from build123d import *

# Parameters (mm, degrees)
SKETCH1_W           = 200
SKETCH1_H           = 150
BOSS_EXTRUDE1_DEPTH = 30
FILLET1_R           = 20
FILLET2_R           = 10
SKETCH2_W           = 15
SKETCH2_H           = 15
CUT_EXTRUDE1_DEPTH  = 183.756668825
FILLET4_R           = 5
SKETCH3_R           = 5
BOSS_EXTRUDE2_DEPTH = 20


with BuildPart() as part:
    # Sketch1 → Boss-Extrude1 (new body)
    with BuildSketch(Plane(origin=(0, 0, 0), x_dir=(1, 0, 0), z_dir=(0, 1, 0))):
        Rectangle(SKETCH1_W, SKETCH1_H)
    extrude(amount=BOSS_EXTRUDE1_DEPTH)

    # Fillet1
    fillet1_edges = [part.edges().sort_by_distance(p)[0] for p in [
        (0, 30, 75),
    ]]
    fillet(fillet1_edges, radius=FILLET1_R)

    # Fillet2
    fillet2_edges = [part.edges().sort_by_distance(p)[0] for p in [
        (100, 30, -10),
        (100, 5, 75),
        (100, 24.142135624, 69.142135624),
        (-100, 5, 75),
        (-100, 24.142135624, 69.142135624),
        (-100, 30, -10),
    ]]
    fillet(fillet2_edges, radius=FILLET2_R)

    # Sketch2 → Cut-Extrude1 (cut, through all)
    with BuildSketch(Plane.XY.offset(75)):
        with Locations((0, 7.5)):
            Rectangle(SKETCH2_W, SKETCH2_H)
    extrude(amount=-CUT_EXTRUDE1_DEPTH, mode=Mode.SUBTRACT)

    # Fillet4
    fillet4_edges = [part.edges().sort_by_distance(p)[0] for p in [
        (-7.5, 0, 0),
        (7.5, 0, 0),
    ]]
    fillet(fillet4_edges, radius=FILLET4_R)

    # Sketch3 → Boss-Extrude2 (add)
    with BuildSketch(Plane(origin=(0, 30, 0), x_dir=(1, 0, 0), z_dir=(0, 1, 0))):
        with Locations(Location((30, 5, 0), (0, 0, 270))):
            Circle(SKETCH3_R)
    boss_extrude2 = extrude(amount=BOSS_EXTRUDE2_DEPTH)

    # Mirror1: Boss-Extrude2 across plane
    add(boss_extrude2.mirror(Plane(origin=(0, 0, 0), x_dir=(0, 0, 1), z_dir=(1, 0, 0))))


solid = part.part
Here's how the part is built. I have some questions about the finished solid (model axes, mm). A direction names the side the tool comes from. Coordinates: 2 decimals unless noted, no trailing zeros. Write each loop counter-clockwise with the first axis right and the second up, starting at its lowest first coordinate (ties: lowest second). Pieces come first, ordered by that corner, then holes.
1) If I drill on line 1 (X direction, y = 7, z = 32.5); line 2 (Y direction, x = -77.5, z = 26.5); line 3 (X direction, y = 2.5, z = -55.5), over which ranges is the centre line in solid material (lowest first)?
Filled in:
line 1: x = -100 to -7.5, 7.5 to 100
line 2: y = 0 to 30
line 3: x = -100 to -8.17, 8.17 to 100
2) Which directions (+Z, -Z, +X, -X, +Y, -Y) give clear straight access to the entire face, cutting with the end or side of a thin tool? Please do faces 4 (the face through (-1, 18, -75)), 5 (the face through (-25.564, 39.86, -2.693)), 6 (the face through (-9, 1.43, -1.05)).
Filled in:
face 4: -Z, +X, -X, +Y, -Y
face 5: +Y
face 6: +Z, -Z, -Y
3) Thinking about a two-plate mould opening in X: for faces 1 (the face through (96.99, 5.07, 72.15)), 2 (the face through (30, 50, -5)), 3 (the face through (25.564, 39.86, -2.693)), which applies, +X half, -X half, draft (parallel to the pull), parting line (faces both ways), or undercut?
Filled in:
face 1: +X half
face 2: draft
face 3: undercut
4) If we section it at A-A (z = -5): List the corners of the cut face in (x, y) for me, plus the area to 3 significant figures.
Filled in:
outline: (-100, 0) - (-12.5, 0) arc R5 ccw to (-7.5, 5) - (-7.5, 15) - (7.5, 15) - (7.5, 5) arc R5 ccw to (12.5, 0) - (100, 0) - (100, 20) arc R10 ccw to (90, 30) - (35, 30) - (35, 50) - (25, 50) - (25, 30) - (-25, 30) - (-25, 50) - (-35, 50) - (-35, 30) - (-90, 30) arc R10 ccw to (-100, 20) - close
area: 6,120 mm2
5) If we section it at D-D (z = 32.5): List the corners of the cut face in (x, y) for me.
Filled in:
outline: (-100, 0) - (-12.5, 0) arc R5 ccw to (-7.5, 5) - (-7.5, 15) - (7.5, 15) - (7.5, 5) arc R5 ccw to (12.5, 0) - (100, 0) - (100, 20) arc R10 ccw to (90, 30) - (-90, 30) arc R10 ccw to (-100, 20) - close
6) If we section it at C-C (x = 47.5): List the corners of the cut face in (y, z) for me, plus the area to 3 significant figures.
Filled in:
outline: (0, -75) - (30, -75) - (30, 55) arc R20 ccw to (10, 75) - (0, 75) - close
area: 4,410 mm2
7) If we section it at B-B (y = 36): List the corners of the cut face in (x, z) for me, plus the area to 3 significant figures.
Filled in:
outline: circle Ø10 at (-30, -5); circle Ø10 at (30, -5)
area: 157 mm2
8) I'm going to push flat-ended pins straight in: pin 1 (1 mm diameter, centred on x = 14.5, z = -18, fed in from +Y); pin 2 (2 mm diameter, centred on x = -11, z = 43, fed in from -Y); pin 3 (8 mm diameter, centred on x = 34.5, y = 42, fed in from -Z). Where does each tip first touch, or does it pass through?
Filled in:
pin 1: stops at y = 30
pin 2: stops at y = 0.03
pin 3: stops at z = -9.97
